The figure shows three views and two pictorial views of one solid part (mm, origin at its lowest corner). Answer the questions. A direction names the side the tool comes from. Coordinates: 2 decimals unless noted, no trailing zeros. Write each loop counter-clockwise with the first axis right and the second up, starting at its lowest first coordinate (ties: lowest second). Pieces come first, ordered by that corner, then holes.
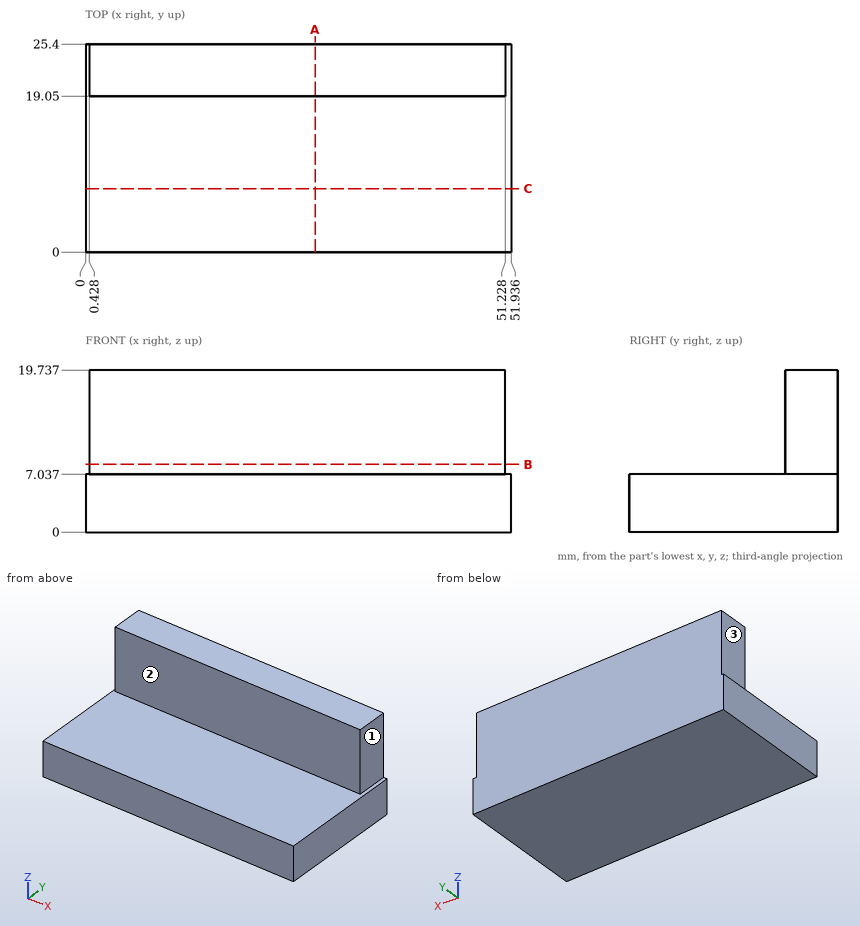
Q1. The part is cut by section C-C, the plane y = 7.75. Write down the section's boundary in (x, z).
Answers below:
outline: (0, 0) - (51.94, 0) - (51.94, 7.04) - (0, 7.04) - close
Q2. Find the intervals of material crossed by probe 1 along Y at (x, z) = (25, 13); probe 2 along Z at (x, y) = (23.5, 3); probe 3 along X at (y, z) = (20.75, 17.75), in increasing order.
Answers below:
probe 1: y = 19.05 to 25.4
probe 2: z = 0 to 7.04
probe 3: x = 0.43 to 51.23
Q3. Given pin 1 (5 mm diameter, centred on y = 23.5, z = 13.5, fed in from +X); pin 2 (7.5 mm diameter, centred on x = 26, y = 9, fed in from +Z); pin 3 (10 mm diameter, centred on x = 25, z = 11, fed in from -Y); pin 4 (7 mm diameter, centred on y = 21.5, z = 14, fed in from -X), each flat-ended and moving along its own axis, determine where each tip first touches the part or whether it passes through.
Answers below:
pin 1: stops at x = 51.23
pin 2: stops at z = 7.04
pin 3: stops at y = 0
pin 4: stops at x = 0.43
Q4. Which of the six approach directions +Z, -Z, +X, -X, +Y, -Y give full straight-line access (tool end or side, diameter ignored) to the marked faces 1, 2 and 3?
Answers below:
face 1: +Z, +X, +Y, -Y
face 2: +Z, +X, -X, -Y
face 3: +Z, -X, +Y, -Y
Q5. The part is cut by section B-B, the plane z = 8.25. Write down the section's boundary in (x, y).
Answers below:
outline: (0.43, 19.05) - (51.23, 19.05) - (51.23, 25.4) - (0.43, 25.4) - close
Q6. The part is cut by section A-A, the plane x = 28. Write down the section's boundary in (y, z).
Answers below:
outline: (0, 0) - (25.4, 0) - (25.4, 19.74) - (19.05, 19.74) - (19.05, 7.04) - (0, 7.04) - close
